Autodesk Inventor part; units mm, degrees
ref_plane "b600_1_XY" through (4.25, 0, 0) normal (1, 0, 0) x (0, 0, -1)
ref_plane "b600_1_YZ" through (4.25, 0, 0) normal (0, 0, -1) x (0, 1, 0)
ref_plane "b600_1_ZX" through (4.25, 0, 0) normal (0, 1, 0) x (1, 0, 0)
sketch "_____1" plane through (0, 0, 0) normal (0, 0, 1) x (1, 0, 0)
  line L0 (5.5, 0) -> (-5.5, 0)
  line L1 (-5.5, 0) -> (-5.5, 7.5)
  line L2 (-5.5, 7.5) -> (5.5, 7.5)
  line L3 (5.5, 7.5) -> (5.5, 0)
  line L4 (5.5, 0) -> (-5.5, 0)
revolve "Revolution1" add sketch "_____1" angle 360 about axis through (5.5, 0, 0) along (1, 0, 0)
sketch "_____3" plane through (0, 0, 0) normal (0, 0, 1) x (1, 0, 0)
  line L0 (5.5, 0) -> (-5.5, 0)
  line L1 (-5.5, 0) -> (-5.5, 4)
  line L2 (-5.5, 4) -> (-3, 4)
  line L3 (-3, 4) -> (-3, 3.5)
  line L4 (-3, 3.5) -> (3, 3.5)
  line L5 (3, 3.5) -> (3, 4)
  line L6 (3, 4) -> (5.5, 4)
  line L7 (5.5, 4) -> (5.5, 0)
  line L8 (5.5, 0) -> (-5.5, 0)
revolve "Revolution2" cut sketch "_____3" angle 360 about axis through (5.5, 0, 0) along (1, 0, 0)
ref_plane "b600_1_XY" through (4.25, 0, 0) normal (1, 0, 0) x (0, 0, -1)
ref_plane "b600_1_YZ" through (4.25, 0, 0) normal (0, 0, -1) x (0, 1, 0)
ref_plane "b600_1_ZX" through (4.25, 0, 0) normal (0, 1, 0) x (1, 0, 0)
ref_plane "b600_2_XY" through (-4.25, 0, 0) normal (1, 0, 0) x (0, 0, -1)
ref_plane "b600_2_YZ" through (-4.25, 0, 0) normal (0, 0, -1) x (0, 1, 0)
ref_plane "b600_2_ZX" through (-4.25, 0, 0) normal (0, 1, 0) x (1, 0, 0)
ref_plane "to_dummy_XY" through (0, 0, 0) normal (1, 0, 0) x (0, 0, -1)
ref_plane "to_dummy_YZ" through (0, 0, 0) normal (0, 0, -1) x (0, 1, 0)
ref_plane "to_dummy_ZX" through (0, 0, 0) normal (0, 1, 0) x (1, 0, 0)
properties part number "C-AFBD11-15_bw"
Input: part model. Units: mm. Frame: model coordinates. A direction names the side the tool comes from. Coordinates: 2 decimals unless noted, no trailing zeros. Loops run counter-clockwise (first coordinate to the right, second up) from the corner with the lowest first, then second, coordinate; pieces in that order, holes last. Notation, with made-up numbers: (-6.75, -4) -> (5.25, -4) arc R18 ccw to (5.25, 7) -> close; hole circle Ø2 at (-4.75, -19). An arc over 180 degrees is marked (long way). Write item = value, one per line. Start each with the question number.
Item 1: Cut plane D-D, the plane z = -6. Return loops of the section in (x, y).
Item 2: Cut plane A-A, the plane y = 0. Return loops of the section in (x, z).
Item 3: Material intervals for line 1 (Z direction, x = 4.1, y = 0); line 2 (Z direction, x = -1.75, y = 0.25); line 3 (Y direction, x = -3.25, z = -2.5), sorted ascending.
Item 4: Cut plane C-C, the plane x = 1.5. Return loops of the section in (y, z), plus the area to 3 significant figures.
Item 5: First-contact query: P1, Ø6, axis at x = -2.5, z = -0.5, coming from the +Y side; P2, Ø1.5, axis at y = 1.5, z = -0.5, coming from the +X side. Flat tips, straight axial feed; report the tip coordinate or a pass-through.
Item 6: Reachability of faces 1 (the face through (5.5, 3, -3)), 2 (the face through (-4.232, -0.867, -3.905)), 3 (the face through (4.268, -0.867, -3.905)) from +Z, -Z, +X, -X, +Y, -Y: full face, straight path, thin tool, end or side. Return the list, or none.
Item 7: Mould query, pull axis Z, two halves, no side actions, for faces 4 (the face through (-5.5, 3, -3)), 5 (the face through (0.077, -7.493, 0.33)), 6 (the face through (0.042, 3.233, -1.341)). Classes: pulls with the +Z half, pulls with the -Z half, needs draft (parallel to the pull), parting line crosses it, or undercut.
Ans:
q1.outline = (-5.5, -4.5) -> (5.5, -4.5) -> (5.5, 4.5) -> (-5.5, 4.5) -> close
q2.outline = (-5.5, -7.5) -> (5.5, -7.5) -> (5.5, -4) -> (3, -4) -> (3, -3.5) -> (-3, -3.5) -> (-3, -4) -> (-5.5, -4) -> close; (-5.5, 4) -> (-3, 4) -> (-3, 3.5) -> (3, 3.5) -> (3, 4) -> (5.5, 4) -> (5.5, 7.5) -> (-5.5, 7.5) -> close
q3.line_1 = -7.5 to -4, 4 to 7.5
q3.line_2 = -7.5 to -3.49, 3.49 to 7.5
q3.line_3 = -7.07 to -3.12, 3.12 to 7.07
q4.outline = circle Ø15 at (0, 0); hole circle Ø7 at (0, 0)
q4.area = 138 mm²
q5.P1 = 7.5
q5.P2 = through
q6.face_1 = +Z, -Z, +X, +Y, -Y
q6.face_2 = -X
q6.face_3 = +X
q7.face_4 = needs draft
q7.face_5 = parting line crosses it
q7.face_6 = undercut
